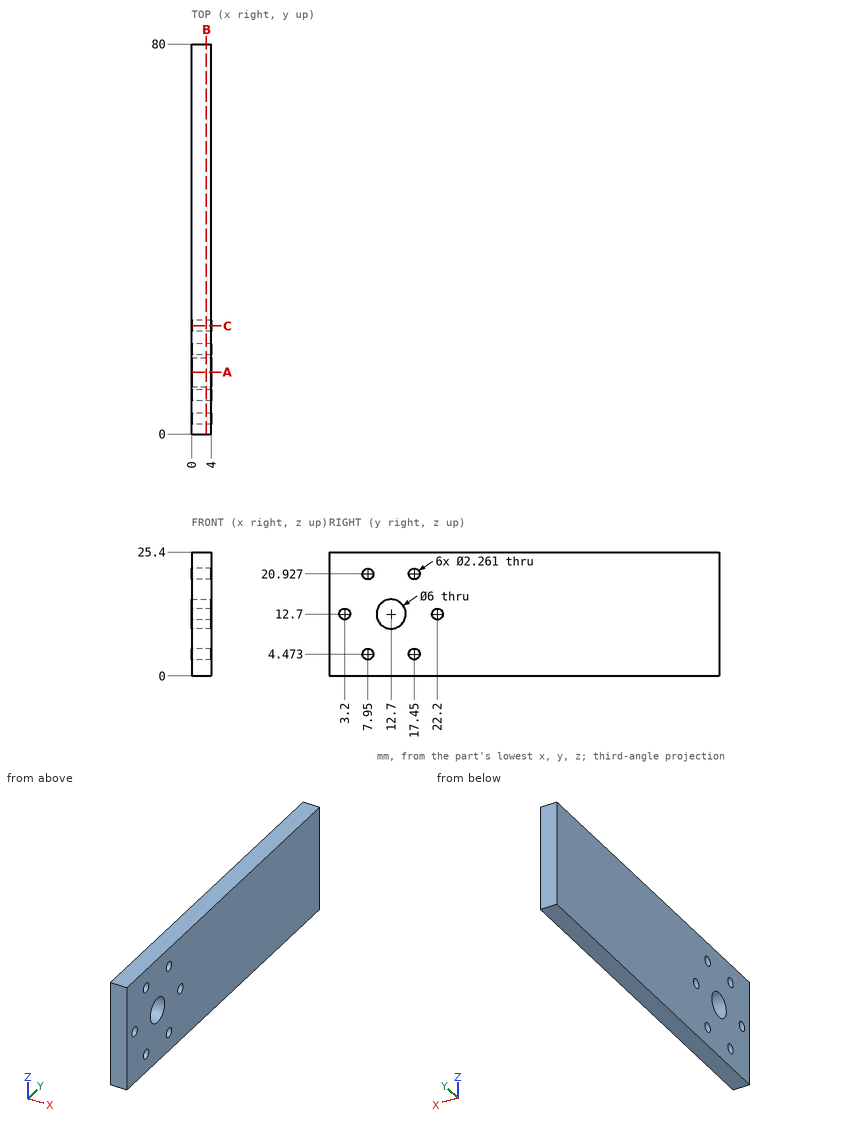
Here's the drawing with two shaded views (mm, measured from the low corner). I have some questions. Round coordinates to 2 decimals unless told otherwise and drop trailing zeros. Loops run counter-clockwise (first coordinate to the right, second up) from the corner with the lowest first, then second, coordinate; pieces in that order, holes last.
Item 1: Suppose I cut it at B-B, the plane x = 3. Write out the boundary of the cut face in (y, z).
Item 2: Suppose I cut it at A-A, the plane y = 12.7. Write out the boundary of the cut face in (x, z), then the cut area to 3 significant figures.
Item 3: Please list where these lines run through material, in increasing order: L1, parallel to Y at x = 2.4, z = 12.7; L2, parallel to Y at x = 1.6, z = 21; L3, parallel to Y at x = 3.7, z = 10.75.
Item 4: Suppose I cut it at C-C, the plane y = 22.2. Write out the boundary of the cut face in (x, z).
Reported:
1. outline: (0, 0) - (80, 0) - (80, 25.4) - (0, 25.4) - close; hole circle Ø2.26 at (3.2, 12.7); hole circle Ø2.26 at (7.95, 4.47); hole circle Ø2.26 at (7.95, 20.93); hole circle Ø6 at (12.7, 12.7); hole circle Ø2.26 at (17.45, 4.47); hole circle Ø2.26 at (17.45, 20.93); hole circle Ø2.26 at (22.2, 12.7)
2. outline: (0, 0) - (4, 0) - (4, 9.7) - (0, 9.7) - close; (0, 15.7) - (4, 15.7) - (4, 25.4) - (0, 25.4) - close
2. area: 77.6 mm2
3. L1: y = 0 to 2.07, 4.33 to 9.7, 15.7 to 21.07, 23.33 to 80
3. L2: y = 0 to 6.82, 9.08 to 16.32, 18.58 to 80
3. L3: y = 0 to 10.42, 14.98 to 80
4. outline: (0, 0) - (4, 0) - (4, 11.57) - (0, 11.57) - close; (0, 13.83) - (4, 13.83) - (4, 25.4) - (0, 25.4) - close
